```python
from build123d import *

# Parameters (mm, degrees)
PAD_DEPTH     = 3
SKETCH001_R   = 31.65
SKETCH001_R_2 = 30.15
PAD001_DEPTH  = 10


with BuildPart() as part:
    # Sketch → Pad (new body)
    with BuildSketch(Plane.XY):
        with BuildLine():
            Line((29.597136, 40), (-29.597136, 40))
            ThreePointArc((-29.597136, 40), (-41.682497, 33.885047), (-43.914336, 20.525875))
            Line((-43.914336, 20.525875), (-28.289336, -29.474125))
            ThreePointArc((-28.289336, -29.474125), (-22.857183, -37.08536), (-13.972136, -40))
            Line((-13.972136, -40), (13.972136, -40))
            ThreePointArc((13.972136, -40), (22.857183, -37.08536), (28.289336, -29.474125))
            Line((28.289336, -29.474125), (43.914336, 20.525875))
            ThreePointArc((43.914336, 20.525875), (41.682497, 33.885047), (29.597136, 40))
        make_face()
    extrude(amount=PAD_DEPTH)

    # Sketch001 (on Face10 of Pad) → Pad001 (join)
    with BuildSketch(Plane.XY.offset(3)):
        Circle(SKETCH001_R)
        Circle(SKETCH001_R_2, mode=Mode.SUBTRACT)
    extrude(amount=PAD001_DEPTH)


solid = part.part
```
Check sheet for the modelled part. Datum: model origin and axes. Units: mm. A direction names the side the tool comes from. Coordinates: 2 decimals unless noted, no trailing zeros. Write each loop counter-clockwise with the first axis right and the second up, starting at its lowest first coordinate (ties: lowest second). Pieces come first, ordered by that corner, then holes. Notation, with made-up numbers: M 41.5,23.25 L 56.5,23.25 A20 cw 56.5,31.25 Z; hole C 41,-18 d7. An arc over 180 degrees is marked long. Use one line per item in the form item = value.
Item 1: Release check for a two-part mould opening along X. For faces 3 (the face through (-6.536, -29.433, 7.93)), 4 (the face through (22.7, -37.2, 1.5)), 5 (the face through (-6.861, -30.897, 7.93)) record: pulls with the +X half, pulls with the -X half, needs draft (parallel to the pull), parting line crosses it, or undercut.
Answer below:
face_3 = undercut
face_4 = pulls with the +X half
face_5 = parting line crosses it
Item 2: Material ranges on L1, parallel to Y at x = 0, z = 8.5; L2, parallel to Z at x = 3.5, y = 35; L3, parallel to Y at x = 12.5, z = 8.25, recorded low to high. Write a range as from..to.
Answer below:
L1 = -31.65..-30.15, 30.15..31.65
L2 = 0..3
L3 = -29.08..-27.44, 27.44..29.08
Item 3: Sectioned sample at A-A, the plane y = 0. Record the cut outline in (x, z), and give its area (3 significant figures).
Answer below:
outline = M -37.5,0 L 37.5,0 L 37.5,3 L 31.65,3 L 31.65,13 L 30.15,13 L 30.15,3 L -30.15,3 L -30.15,13 L -31.65,13 L -31.65,3 L -37.5,3 Z
area = 255 mm^2
Item 4: Sectioned sample at B-B, the plane z = 2. Record the cut outline in (x, y).
Answer below:
outline = M -43.91,20.53 L -28.29,-29.47 A15 ccw -13.97,-40 L 13.97,-40 A15 ccw 28.29,-29.47 L 43.91,20.53 A15 ccw 29.6,40 L -29.6,40 A15 ccw Z
Item 5: Sectioned sample at C-C, the plane x = 0. Record the cut outline in (y, z), and give its area (3 significant figures).
Answer below:
outline = M -40,0 L 40,0 L 40,3 L 31.65,3 L 31.65,13 L 30.15,13 L 30.15,3 L -30.15,3 L -30.15,13 L -31.65,13 L -31.65,3 L -40,3 Z
area = 270 mm^2
Item 6: Set-up check for faces 1 (the face through (0, 40, 1)), 2 (the face through (0, 0, 3)): record each of +Z, -Z, +X, -X, +Y, -Y from which the full face is reachable in a straight line by a thin tool's end or side.
Answer below:
face_1 = +Z, -Z, +X, -X, +Y
face_2 = +Z
Item 7: Gauge pin test, flat ends, axial feed: pin 1 Ø6 at (x, z) = (23.5, 3) entering from -Y; pin 2 Ø1 at (x, z) = (14, 10.5) entering from -Y; pin 3 Ø5 at (x, y) = (-11.5, 7.5) entering from +Z; pin 4 Ø3 at (x, y) = (34.5, 9) entering from -Z. Record the tip position at first contact, or that the pin passes through.
Answer below:
pin_1 = -38.51
pin_2 = -28.63
pin_3 = 3
pin_4 = 0
